Could you check a few things on this model? Use its own coordinates, in mm. Face numbers are marked on the shaded views. A direction names the side the tool comes from. Round coordinates to 2 decimals unless told otherwise and drop trailing zeros. Loops run counter-clockwise (first coordinate to the right, second up) from the corner with the lowest first, then second, coordinate; pieces in that order, holes last. Notation, with made-up numbers: (-11, 11) - (7, 11) arc R20 cw to (7, 37) - close; hole circle Ø4 at (87, 24.5). An arc over 180 degrees is marked (long way). Use one line per item in the form item = value.
```python
from build123d import *

# Parameters (mm, degrees)
SKETCH_R        = 2.75
SKETCH_R_2      = 8.1
PAD_DEPTH       = 10
SKETCH001_R     = 14
SKETCH001_R_2   = 8.1
PAD001_DEPTH    = 32
CHAMFER_SIZE    = 0.5
FILLET_R        = 0.5
CHAMFER001_SIZE = 0.5
POCKET_DEPTH    = 10


with BuildPart() as part:
    # Sketch → Pad (new body)
    with BuildSketch(Plane.YZ):
        with BuildLine():
            ThreePointArc((-13.266499, 20), (-24, 0), (-13.266499, -20))
            Line((-13.266499, -20), (13.266499, -20))
            ThreePointArc((13.266499, -20), (24, 0), (13.266499, 20))
            Line((-13.266499, 20), (13.266499, 20))
        make_face()
        with Locations((-13.435058, 13.435)):
            Circle(SKETCH_R, mode=Mode.SUBTRACT)
        with Locations((-19, 0)):
            Circle(SKETCH_R, mode=Mode.SUBTRACT)
        with Locations((-13.435058, -13.435)):
            Circle(SKETCH_R, mode=Mode.SUBTRACT)
        with Locations((13.435058, 13.435)):
            Circle(SKETCH_R, mode=Mode.SUBTRACT)
        with Locations((19, 0)):
            Circle(SKETCH_R, mode=Mode.SUBTRACT)
        with Locations((13.435058, -13.435)):
            Circle(SKETCH_R, mode=Mode.SUBTRACT)
        Circle(SKETCH_R_2, mode=Mode.SUBTRACT)
    extrude(amount=PAD_DEPTH)

    # Sketch001 → Pad001 (new body)
    with BuildSketch(Plane.YZ.offset(10)):
        Circle(SKETCH001_R)
        Circle(SKETCH001_R_2, mode=Mode.SUBTRACT)
    extrude(amount=PAD001_DEPTH)

    # Chamfer
    chamfer_edges = [part.edges().sort_by_distance(p)[0] for p in [
        (0, -16.185058, -13.435),
        (10, -16.185058, -13.435),
        (0, -21.75, 0),
        (10, -21.75, 0),
        (0, -16.185058, 13.435),
        (10, -16.185058, 13.435),
        (0, 10.685058, 13.435),
        (10, 10.685058, 13.435),
        (0, 16.25, 0),
        (10, 16.25, 0),
        (0, 10.685058, -13.435),
        (10, 10.685058, -13.435),
    ]]
    chamfer(chamfer_edges, length=CHAMFER_SIZE)

    # Fillet
    fillet_edges = [part.edges().sort_by_distance(p)[0] for p in [
        (42, -14, 0),
    ]]
    fillet(fillet_edges, radius=FILLET_R)

    # Chamfer001
    chamfer001_edges = [part.edges().sort_by_distance(p)[0] for p in [
        (5, -13.266499, 20),
        (5, -13.266499, -20),
        (0, -24, 0),
        (10, -24, 0),
        (5, 13.266499, 20),
        (0, 0, 20),
        (10, 0, 20),
        (5, 13.266499, -20),
        (0, 24, 0),
        (10, 24, 0),
        (0, 0, -20),
        (10, 0, -20),
    ]]
    chamfer(chamfer001_edges, length=CHAMFER001_SIZE)

    # Sketch002 → Pocket (cut)
    with BuildSketch(Plane(origin=(0, 0, 0), x_dir=(0, 1, 0), z_dir=(-1, 0, 0))):
        with BuildLine():
            ThreePointArc((-9.970206, 9.970206), (-14.1, 0), (-9.970206, -9.970206))
            Line((-9.970206, -9.970206), (-2.737206, -20.3))
            Line((-2.737206, -20.3), (18, -20.3))
            Line((18, -20.3), (18, -27))
            Line((18, -27), (0, -27))
            ThreePointArc((0, 27), (-27, 0), (0, -27))
            Line((0, 27), (18, 27))
            Line((18, 27), (18, 20.3))
            Line((18, 20.3), (-2.737206, 20.3))
            Line((-9.970206, 9.970206), (-2.737206, 20.3))
        make_face()
    extrude(amount=-POCKET_DEPTH, mode=Mode.SUBTRACT)


solid = part.part
```
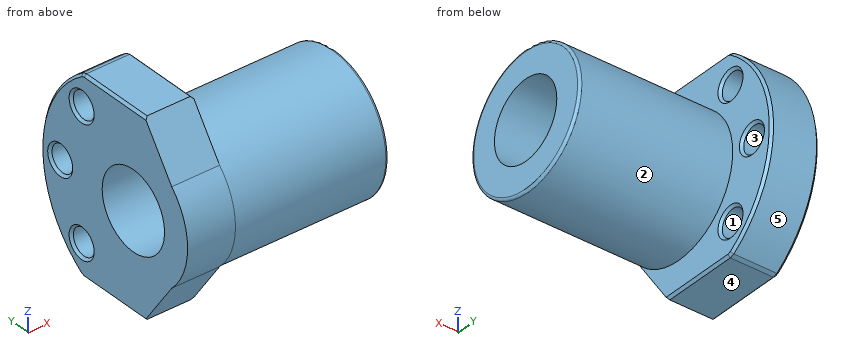
1. For P1, Ø3, axis at x = 22.5, z = -4, coming from the +Y side (3 decimals); P2, Ø8, axis at x = 23.5, y = 15, coming from the +Z side; P3, Ø2, axis at x = 35.5, z = -12.5, coming from the +Y side; P4, Ø5, axis at y = 19, z = 0, coming from the +X side, each with a flat end and sliding along its axis, tell me the tip position at first contact or that it passes through.
Solution:
P1 = 13.775
P2 = 8.66
P3 = 7.98
P4 = through
2. On a 3-axis mill with a long thin cutter (end or side, diameter ignored), from which of +Z, -Z, +X, -X, +Y, -Y can I reach the whole of each face in a straight line? I mean the marked faces 1 and 2. Say none if no direction works.
Solution:
face_1 = +X, -X
face_2 = +X
3. If we section it at B-B, the plane z = 0: Write out the boundary of the cut face in (x, y).
Solution:
outline = (0, -14.1) - (10, -14.1) - (10, -14) - (41.5, -14) arc R0.5 ccw to (42, -13.5) - (42, -8.1) - (0, -8.1) - close; (0, 8.1) - (42, 8.1) - (42, 13.5) arc R0.5 ccw to (41.5, 14) - (10, 14) - (10, 15.75) - (9.5, 16.25) - (0.5, 16.25) - (0, 15.75) - close; (0, 22.25) - (0.5, 21.75) - (9.5, 21.75) - (10, 22.25) - (10, 23.5) - (9.5, 24) - (0.5, 24) - (0, 23.5) - close
4. We'd pull the mould along Z, two halves only. Please class the marked faces 3, 4 and 5: +Z half, -Z half, draft (parallel to the pull), parting line (faces both ways), or undercut.
Solution:
face_3 = undercut
face_4 = -Z half
face_5 = parting line
5. If we section it at C-C, the plane x = 33: Write out the boundary of the cut face in (y, z), plus the area to 3 significant figures.
Solution:
outline = circle Ø28 at (0, 0); hole circle Ø16.2 at (0, 0)
area = 410 mm^2
6. Please list where these lines run through material, in increasing order: line 1 along Y through (x, z) = (3.5, 2.5); line 2 along Z through (x, y) = (9.5, 11.5); line 3 along X through (y, z) = (22, 7).
Solution:
line_1 = -13.88 to -7.7, 7.7 to 17.85, 20.15 to 23.87
line_2 = -20 to -15.39, -11.48 to 11.48, 15.39 to 20
line_3 = 0 to 10
7. If we section it at A-A, the plane y = 0: Write out the boundary of the cut face in (x, z), plus the area to 3 significant figures.
Solution:
outline = (0, -19.5) - (0.5, -20) - (9.5, -20) - (10, -19.5) - (10, -14) - (41.5, -14) arc R0.5 ccw to (42, -13.5) - (42, -8.1) - (0, -8.1) - close; (0, 8.1) - (42, 8.1) - (42, 13.5) arc R0.5 ccw to (41.5, 14) - (10, 14) - (10, 19.5) - (9.5, 20) - (0.5, 20) - (0, 19.5) - close
area = 615 mm^2
